Design review of the part shown in the three views and the two pictorial views. Dimensions are in mm from the part's minimum x, y and z. A direction names the side the tool comes from. Round coordinates to 2 decimals unless told otherwise and drop trailing zeros. Loops run counter-clockwise (first coordinate to the right, second up) from the corner with the lowest first, then second, coordinate; pieces in that order, holes last. Notation, with made-up numbers: M -10.75,20.25 L 7.25,20.25 A5 cw 7.25,24.25 Z; hole C -12,30.25 d4. An arc over 180 degrees is marked long. One line per question, with ' | ' between items. Start each with the question number.
1) For the marked faces 1, 2 and 3, list the 3-axis set-ups (+Z, -Z, +X, -X, +Y, -Y) from which the entire face can be reached by the end or side of a thin tool; tool diameter is ignored.
2) We need section C-C (z = 61). Give the boundary of the cut face in (x, y), and give its area (3 significant figures).
3) We need section A-A (y = 13). Give the boundary of the cut face in (x, z).
4) For pin 1 Ø4 at (x, y) = (21, 20.5) entering from -Z; pin 2 Ø2 at (y, z) = (19.5, 31) entering from +X; pin 3 Ø2 at (x, z) = (14, 29.5) entering from -Y, all flat-tipped, find the tip position at first contact; note any pin that passes through.
5) For probe 1 along Z at (x, y) = (7.5, 22.5); probe 2 along Z at (x, y) = (20.5, 17.5); probe 3 along Y at (x, z) = (12.25, 77.5), list the stretches that pass through material, from the lowest coordinate up. Write a range as from..to.
6) We need section D-D (z = 23). Give the boundary of the cut face in (x, y).
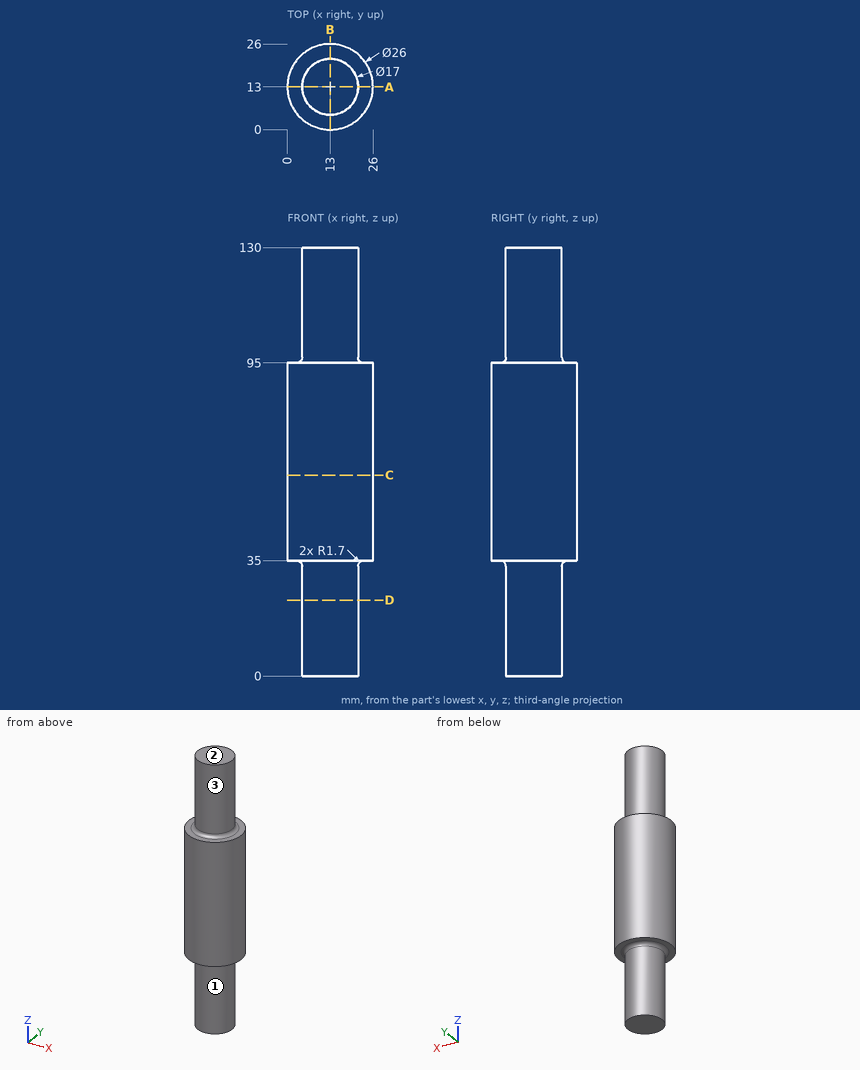
Answers below:
1) face 1: -Z | face 2: +Z, +X, -X, +Y, -Y | face 3: +Z
2) outline: C 13,13 d26 | area: 531 mm^2
3) outline: M 0,35 L 2.8,35 A1.7 cw 4.5,33.3 L 4.5,0 L 21.5,0 L 21.5,33.3 A1.7 cw 23.2,35 L 26,35 L 26,95 L 23.2,95 A1.7 cw 21.5,96.7 L 21.5,130 L 4.5,130 L 4.5,96.7 A1.7 cw 2.8,95 L 0,95 Z
4) pin 1: z = 34.47 | pin 2: x = 19.48 | pin 3: y = 4.5
5) probe 1: 35..95 | probe 2: 34.18..95.82 | probe 3: 0.02..25.98
6) outline: C 13,13 d17
